Verification items for the finished model (mm, model axes). Coordinates: 2 decimals unless noted, no trailing zeros. Write each loop counter-clockwise with the first axis right and the second up, starting at its lowest first coordinate (ties: lowest second). Pieces come first, ordered by that corner, then holes. Notation, with made-up numbers: (11.5, 49) -> (24.5, 49) arc R14 ccw to (24.5, 76) -> close; hole circle Ø3 at (-3.75, 84.25). An arc over 180 degrees is marked (long way). Answer in a Markdown table with one row per item.
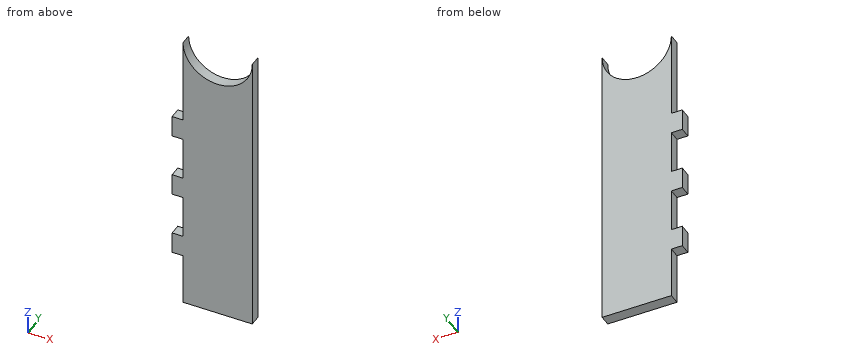
```python
from build123d import *

# Parameters (mm, degrees)
BOSS_EXTRUDE1_DEPTH = 5


with BuildPart() as part:
    # Sketch9 → Boss-Extrude1 (new body)
    with BuildSketch(Plane(origin=(0, 0, 0), x_dir=(1, 0, 0), z_dir=(0, 1, 0))):
        with BuildLine():
            Line((-15.875, 109.875), (-15.875, 133.875))
            Line((-15.875, 133.875), (15.875, 133.875))
            Line((15.875, 133.875), (15.875, 0))
            ThreePointArc((15.875, 0), (0, 15.875), (-15.875, 0))
            Line((-15.875, 0), (-15.875, 39.875))
            Line((-15.875, 39.875), (-20.875, 39.875))
            Line((-20.875, 39.875), (-20.875, 49.875))
            Line((-20.875, 49.875), (-15.875, 49.875))
            Line((-15.875, 49.875), (-15.875, 69.875))
            Line((-15.875, 69.875), (-20.875, 69.875))
            Line((-20.875, 69.875), (-20.875, 79.875))
            Line((-20.875, 79.875), (-15.875, 79.875))
            Line((-15.875, 79.875), (-15.875, 99.875))
            Line((-15.875, 99.875), (-20.875, 99.875))
            Line((-20.875, 99.875), (-20.875, 109.875))
            Line((-20.875, 109.875), (-15.875, 109.875))
        make_face()
    extrude(amount=BOSS_EXTRUDE1_DEPTH)


solid = part.part
```
1. Section check D-D, the plane x = -12. Record the boundary of the cut face in (y, z) (3 decimals), plus the area to 3 significant figures.
Geometry says:
| item | result |
|---|---|
| outline | (0, -133.875) -> (5, -133.875) -> (5, -10.393) -> (0, -10.393) -> close |
| area | 617 mm^2 |
2. Depth check by flat-ended pin: P1, Ø3, axis at y = 4, z = -21.5, coming from the -X side (3 decimals). Enter the tip coordinate at first touch or a pass-through.
Geometry says:
| item | result |
|---|---|
| P1 | x = -15.875 |
3. Section check C-C, the plane x = 0. Record the boundary of the cut face in (y, z) (3 decimals).
Geometry says:
| item | result |
|---|---|
| outline | (0, -133.875) -> (5, -133.875) -> (5, -15.875) -> (0, -15.875) -> close |
4. Thickness scan on line 1 (Z direction, x = -19, y = 1.7) (3 decimals); line 2 (X direction, y = 1.15, z = -97) (3 decimals); line 3 (X direction, y = 3.1, z = -12) (3 decimals). Record the ranges inside material, lowest first. Write a range as from..to.
Geometry says:
| item | result |
|---|---|
| line 1 | -109.875..-99.875, -79.875..-69.875, -49.875..-39.875 |
| line 2 | -15.875..15.875 |
| line 3 | -15.875..-10.393, 10.393..15.875 |
5. Section check A-A, the plane y = 4.25. Record the boundary of the cut face in (x, z) (3 decimals), plus the area to 3 significant figures.
Geometry says:
| item | result |
|---|---|
| outline | (-20.875, -109.875) -> (-15.875, -109.875) -> (-15.875, -133.875) -> (15.875, -133.875) -> (15.875, 0) arc R15.875 cw to (-15.875, 0) -> (-15.875, -39.875) -> (-20.875, -39.875) -> (-20.875, -49.875) -> (-15.875, -49.875) -> (-15.875, -69.875) -> (-20.875, -69.875) -> (-20.875, -79.875) -> (-15.875, -79.875) -> (-15.875, -99.875) -> (-20.875, -99.875) -> close |
| area | 4,000 mm^2 |
6. Section check B-B, the plane z = -13.5. Record the boundary of the cut face in (x, y) (3 decimals), plus the area to 3 significant figures.
Geometry says:
| item | result |
|---|---|
| outline | (-15.875, 0) -> (-8.353, 0) -> (-8.353, 5) -> (-15.875, 5) -> close; (8.353, 0) -> (15.875, 0) -> (15.875, 5) -> (8.353, 5) -> close |
| area | 75.2 mm^2 |
